Check sheet for the modelled part. Datum: model origin and axes. Units: mm. Face numbers are marked on the shaded views. A direction names the side the tool comes from. Give positions to 0.01 mm unless a question says otherwise; leave off trailing zeros. Loops run counter-clockwise (first coordinate to the right, second up) from the corner with the lowest first, then second, coordinate; pieces in that order, holes last. Notation, with made-up numbers: (12.25, 49) - (43.25, 49) arc R7 cw to (43.25, 55) - close; hole circle Ø7 at (9.25, 30). An arc over 180 degrees is marked (long way). Use one line per item in the form item = value.
from build123d import *

# Parameters (mm, degrees)
SKETCH3_R      = 6.35
SKETCH5_R      = 6.8961
SKETCH7_R      = 5.0165
EXTRUDE2_DEPTH = 20.066


with BuildPart() as part:
    # Sketch2 → Revolve1 (revolve)
    with BuildSketch(Plane.XY, mode=Mode.PRIVATE) as revolve1_sk:
        Polygon((18.415, 1.9685), (20.447, 1.9685), (21.209, 2.7305), (21.209, 8.509), (8.5979, 8.509), (8.5979, 1.524), (8.5979, 0), (10.287, 0), (10.287, 1.4478), (18.415, 1.4478), align=None)
    revolve(revolve1_sk.sketch.rotate(Axis((21.209, 8.509, 0), (-1, 0, 0)), 270), axis=Axis((21.209, 8.509, 0), (-1, 0, 0)))

    # Sketch3 → Loft2 section 0
    with BuildSketch(Plane(origin=(0, 0, 0), x_dir=(0, 0, -1), z_dir=(1, 0, 0))):
        with Locations((0, 8.509)):
            Circle(SKETCH3_R)
    # Sketch5 → Loft2 section 1
    with BuildSketch(Plane(origin=(8.636, 0, 0), x_dir=(0, 0, -1), z_dir=(1, 0, 0))):
        with Locations((0, 8.509)):
            Circle(SKETCH5_R)
    loft()

    # Sketch7 → Extrude2 (cut)
    with BuildSketch(Plane(origin=(21.209, 0, 0), x_dir=(0, 0, -1), z_dir=(1, 0, 0))):
        with Locations((0, 8.509)):
            Circle(SKETCH7_R)
    extrude(amount=-EXTRUDE2_DEPTH, mode=Mode.SUBTRACT)


solid = part.part
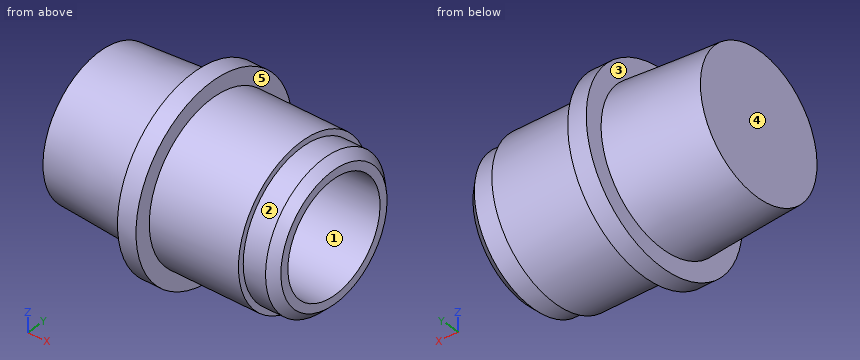
Item 1: Thickness scan on L1, parallel to Y at x = 15, z = 0; L2, parallel to X at y = 4.5, z = 7; L3, parallel to Y at x = 13, z = 2.5. Record the ranges inside material, lowest first.
Answer block:
L1 = 1.45 to 3.49, 13.53 to 15.57
L2 = 8.6 to 10.29
L3 = 1.91 to 4.16, 12.86 to 15.11
Item 2: Section check A-A on z = 0. Record the boundary of the cut face in (x, y) (1 decimal).
Answer block:
outline = (0, 2.2) - (8.6, 1.6) - (8.6, 0) - (10.3, 0) - (10.3, 1.4) - (18.4, 1.4) - (18.4, 2) - (20.4, 2) - (21.2, 2.7) - (21.2, 3.5) - (1.1, 3.5) - (1.1, 13.5) - (21.2, 13.5) - (21.2, 14.3) - (20.4, 15) - (18.4, 15) - (18.4, 15.6) - (10.3, 15.6) - (10.3, 17) - (8.6, 17) - (8.6, 15.4) - (0, 14.9) - close
Item 3: Access from +Z, -Z, +X, -X, +Y, -Y to the whole of each face (thin tool, end or side, straight path). Record for the marked faces 4 and 5.
Answer block:
face_4 = +Z, -Z, -X, +Y, -Y
face_5 = +X
Item 4: Mould release check, pull along Z, two halves, no side actions. Record for the marked faces 1, 2 and 3: released by +Z, released by -Z, zero draft, split by the parting line, or undercut.
Answer block:
face_1 = undercut
face_2 = split by the parting line
face_3 = zero draft
Item 5: Section check C-C on x = 18.75. Record the boundary of the cut face in (y, z), then the cut area to 3 significant figures.
Answer block:
outline = circle Ø13.08 at (8.51, 0); hole circle Ø10.03 at (8.51, 0)
area = 55.3 mm2
Item 6: Section check B-B on x = 16. Record the boundary of the cut face in (y, z).
Answer block:
outline = circle Ø14.12 at (8.51, 0); hole circle Ø10.03 at (8.51, 0)
Item 7: Gauge pin test, flat ends, axial feed: P1, Ø8, axis at x = 14.5, y = 2.5, coming from the -Z side; P2, Ø4, axis at x = 13.5, y = 5, coming from the -Z side; P3, Ø8, axis at x = 2.5, z = 6.5, coming from the +Y side. Record the tip position at first contact, or that the pin passes through.
Answer block:
P1 = -6.77
P2 = -6.9
P3 = 14.54
